from build123d import *

# Parameters (mm, degrees)
SKETCH1_W           = 20.066
SKETCH1_H           = 50.8
BOSS_EXTRUDE1_DEPTH = 12.7
SKETCH2_R           = 2.286
CUT_EXTRUDE1_DEPTH  = 13.7
SKETCH3_W           = 40
SKETCH3_H           = 50.8
BOSS_EXTRUDE2_DEPTH = 6.35
SKETCH5_R           = 1.75
CUT_EXTRUDE2_DEPTH  = 7.35
SKETCH6_R           = 6.35
CUT_EXTRUDE3_DEPTH  = 6.35
FILLET1_R           = 6.35


with BuildPart() as part:
    # Sketch1 → Boss-Extrude1 (new body)
    with BuildSketch(Plane.XY):
        Rectangle(SKETCH1_W, SKETCH1_H)
    extrude(amount=BOSS_EXTRUDE1_DEPTH)

    # Sketch2 → Cut-Extrude1 (cut, through all)
    with BuildSketch(Plane.XY.offset(12.7)):
        with Locations((0, 12.7)):
            Circle(SKETCH2_R)
        with Locations((0, -12.7)):
            Circle(SKETCH2_R)
    extrude(amount=-CUT_EXTRUDE1_DEPTH, mode=Mode.SUBTRACT)

    # Sketch3 → Boss-Extrude2 (add)
    with BuildSketch(Plane.XY.offset(12.7)):
        with Locations((-30.033, 0)):
            Rectangle(SKETCH3_W, SKETCH3_H)
    extrude(amount=-BOSS_EXTRUDE2_DEPTH)

    # Sketch5 → Cut-Extrude2 (cut, through all)
    with BuildSketch(Plane(origin=(0, 0, 6.35), x_dir=(-1, 0, 0), z_dir=(0, 0, -1))):
        with Locations((43.033, 8.5)):
            Circle(SKETCH5_R)
        with Locations((17.033, 8.5)):
            Circle(SKETCH5_R)
        with Locations((43.033, -8.5)):
            Circle(SKETCH5_R)
        with Locations((17.033, -8.5)):
            Circle(SKETCH5_R)
    extrude(amount=-CUT_EXTRUDE2_DEPTH, mode=Mode.SUBTRACT)

    # Sketch6 → Cut-Extrude3 (cut)
    with BuildSketch(Plane.XY.offset(12.7)):
        with Locations((0, 12.7)):
            Circle(SKETCH6_R)
        with Locations((0, -12.7)):
            Circle(SKETCH6_R)
    extrude(amount=-CUT_EXTRUDE3_DEPTH, mode=Mode.SUBTRACT)

    # Fillet1
    fillet1_edges = [part.edges().sort_by_distance(p)[0] for p in [
        (-50.033, -25.4, 9.525),
        (-50.033, 25.4, 9.525),
        (10.033, -25.4, 6.35),
        (10.033, 25.4, 6.35),
    ]]
    fillet(fillet1_edges, radius=FILLET1_R)


solid = part.part
Here's how the part is built. I have some questions about the finished solid (model axes, mm). A direction names the side the tool comes from. Coordinates: 2 decimals unless noted, no trailing zeros. Order: outer loops, then holes, each group sorted by start corner. A loop starts at its lowest first (then second) coordinate and runs counter-clockwise, first axis right, second up.
Item 1: If we section it at C-C on y = -12.7: List the corners of the cut face in (x, z) for me.
Result sheet:
outline: (-50.03, 6.35) - (-10.03, 6.35) - (-10.03, 0) - (-2.29, 0) - (-2.29, 6.35) - (-6.35, 6.35) - (-6.35, 12.7) - (-50.03, 12.7) - close; (2.29, 0) - (10.03, 0) - (10.03, 12.7) - (6.35, 12.7) - (6.35, 6.35) - (2.29, 6.35) - close
Item 2: If we section it at B-B on z = 10.75: List the corners of the cut face in (x, y) for me, plus the area to 3 significant figures.
Result sheet:
outline: (-50.03, -19.05) arc R6.35 ccw to (-43.68, -25.4) - (3.68, -25.4) arc R6.35 ccw to (10.03, -19.05) - (10.03, 19.05) arc R6.35 ccw to (3.68, 25.4) - (-43.68, 25.4) arc R6.35 ccw to (-50.03, 19.05) - close; hole circle Ø3.5 at (-43.03, -8.5); hole circle Ø3.5 at (-43.03, 8.5); hole circle Ø3.5 at (-17.03, -8.5); hole circle Ø3.5 at (-17.03, 8.5); hole circle Ø12.7 at (0, -12.7); hole circle Ø12.7 at (0, 12.7)
area: 2,720 mm2
Item 3: If we section it at D-D on y = 8.5: List the corners of the cut face in (x, z) for me, plus the area to 3 significant figures.
Result sheet:
outline: (-50.03, 6.35) - (-44.78, 6.35) - (-44.78, 12.7) - (-50.03, 12.7) - close; (-41.28, 6.35) - (-18.78, 6.35) - (-18.78, 12.7) - (-41.28, 12.7) - close; (-15.28, 6.35) - (-10.03, 6.35) - (-10.03, 0) - (10.03, 0) - (10.03, 12.7) - (4.76, 12.7) - (4.76, 6.35) - (-4.76, 6.35) - (-4.76, 12.7) - (-15.28, 12.7) - close
area: 404 mm2
Item 4: For faces 5 (the face through (3, 13, 6.35)), 6 (the face through (-30, 0, 6.35)), 7 (the face through (-15, -25.4, 8)), which set-ups out of +Z, -Z, +X, -X, +Y, -Y let a thin tool reach every point of the face, with its end or its side?
Result sheet:
face 5: +Z
face 6: -Z, -X, +Y, -Y
face 7: +Z, -Z, +X, -X, -Y
Item 5: If we mould it in two halves opening along X, with no side actions, what happens to faces 1 (the face through (-10.033, 0, 3)), 2 (the face through (10.033, 0, 6)), 3 (the face through (3, -13, 6.35)), 4 (the face through (-20, 0, 12.7))? For each: +X half, -X half, draft (parallel to the pull), parting line (faces both ways), or undercut.
Result sheet:
face 1: -X half
face 2: +X half
face 3: undercut
face 4: draft
Item 6: For P1, Ø10, axis at x = -3, y = -11, coming from the +Z side; P2, Ø2, axis at x = -43.033, y = -8.5, coming from the -Z side; P3, Ø5.5, axis at x = -17.033, y = 8.5, coming from the -Z side; P4, Ø1.9, axis at y = -1.5, z = 4, coming from the -X side, each with a flat end and sliding along its axis, tell me the tip position at first contact or that it passes through.
Result sheet:
P1: stops at z = 12.7
P2: passes through
P3: stops at z = 6.35
P4: stops at x = -10.03
Item 7: If we section it at A-A on x = 0: List the corners of the cut face in (y, z) for me.
Result sheet:
outline: (-25.4, 0) - (-14.99, 0) - (-14.99, 6.35) - (-19.05, 6.35) - (-19.05, 12.7) - (-25.4, 12.7) - close; (-10.41, 0) - (10.41, 0) - (10.41, 6.35) - (6.35, 6.35) - (6.35, 12.7) - (-6.35, 12.7) - (-6.35, 6.35) - (-10.41, 6.35) - close; (14.99, 0) - (25.4, 0) - (25.4, 12.7) - (19.05, 12.7) - (19.05, 6.35) - (14.99, 6.35) - close
Item 8: I need wall thicknesses on line 1 (Y direction, x = -0.5, z = 11.75); line 2 (X direction, y = 8, z = 9.25); line 3 (X direction, y = 17, z = 3.75). Which ranges of each line are inside material? Lowest first, please.
Result sheet:
line 1: y = -25.4 to -19.03, -6.37 to 6.37, 19.03 to 25.4
line 2: x = -50.03 to -44.71, -41.36 to -18.71, -15.36 to -4.27, 4.27 to 10.03
line 3: x = -10.03 to 10.03
